Job drawing, mm, ordinate dimensions from the low corner. One solid piece. Round coordinates to 2 decimals unless told otherwise and drop trailing zeros. Loops run counter-clockwise (first coordinate to the right, second up) from the corner with the lowest first, then second, coordinate; pieces in that order, holes last. Notation, with made-up numbers: M 50.25,5.25 L 101.25,5.25 A20 cw 101.25,40.25 Z; hole C 51.25,87 d9. An arc over 180 degrees is marked long. Put each result on its own line as item: value. Start each with the question number.
1) Slice it at A-A on z = 19.25. Give the cut face in (x, y) (1 decimal).
2) Probe line 1 along X through (y, z) = (1.2, 19.25) (1 decimal); line 2 along X through (y, z) = (0.45, 5.5) (1 decimal); line 3 along X through (y, z) = (0.8, 3.5). List the from-to ranges inside material, lowest first.
3) Drop a flat-ended pin along its axis: pin 1 Ø1.2 at (x, z) = (6.19, 3.25) entering from +Y. Give the stop position or say it passes through.
4) Slice it at B-B on x = 30. Give the cut face in (y, z) (1 decimal).
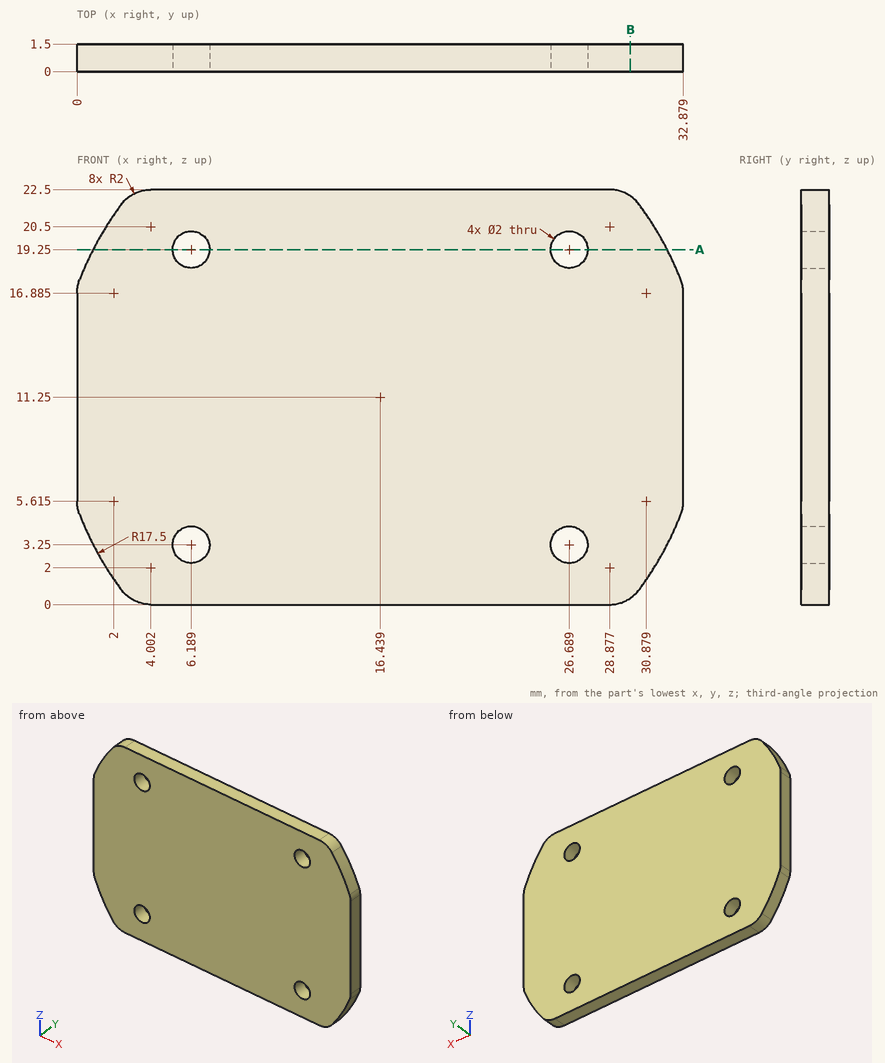
Recorded:
1. outline: M 0.9,0 L 5.2,0 L 5.2,1.5 L 0.9,1.5 Z; M 7.2,0 L 25.7,0 L 25.7,1.5 L 7.2,1.5 Z; M 27.7,0 L 32,0 L 32,1.5 L 27.7,1.5 Z
2. line 1: x = 0.9 to 5.2, 7.2 to 25.7, 27.7 to 32
2. line 2: x = 0 to 32.9
2. line 3: x = 0.75 to 5.22, 7.16 to 25.72, 27.66 to 32.13
3. pin 1: passes through
4. outline: M 0,0.3 L 1.5,0.3 L 1.5,22.2 L 0,22.2 Z
